from build123d import *

# Parameters (mm, degrees)
SKETCH2_R           = 7
SKETCH2_R_2         = 4
BOSS_EXTRUDE1_DEPTH = 2
SKETCH3_R           = 6.5
SKETCH3_R_2         = 4.5
CUT_EXTRUDE1_DEPTH  = 0.25
FILLET1_R           = 0.25
CHAMFER1_SIZE       = 0.125


with BuildPart() as part:
    # Sketch2 → Boss-Extrude1 (new body, symmetric)
    with BuildSketch(Plane(origin=(0, 0, 0), x_dir=(1, 0, 0), z_dir=(0, 1, 0))):
        Circle(SKETCH2_R)
        Circle(SKETCH2_R_2, mode=Mode.SUBTRACT)
    extrude(amount=BOSS_EXTRUDE1_DEPTH, both=True)

    # Sketch3 → Cut-Extrude1 (cut)
    with BuildSketch(Plane(origin=(0, 2, 0), x_dir=(1, 0, 0), z_dir=(0, 1, 0))):
        Circle(SKETCH3_R)
        Circle(SKETCH3_R_2, mode=Mode.SUBTRACT)
    cut_extrude1 = extrude(amount=-CUT_EXTRUDE1_DEPTH, mode=Mode.SUBTRACT)

    # Mirror1: Cut-Extrude1 across plane
    add(cut_extrude1.mirror(Plane.ZX), mode=Mode.SUBTRACT)

    # Fillet1
    fillet1_edges = [part.edges().sort_by_distance(p)[0] for p in [
        (-7, -2, 0),
        (-7, 2, 0),
    ]]
    fillet(fillet1_edges, radius=FILLET1_R)

    # Chamfer1
    chamfer1_edges = [part.edges().sort_by_distance(p)[0] for p in [
        (-4, -2, 0),
        (-4, 2, 0),
    ]]
    chamfer(chamfer1_edges, length=CHAMFER1_SIZE)


solid = part.part
Design review of the part built by this model. Coordinates are the model's own, in mm. A direction names the side the tool comes from. Coordinates: 2 decimals unless noted, no trailing zeros. Loops run counter-clockwise (first coordinate to the right, second up) from the corner with the lowest first, then second, coordinate; pieces in that order, holes last. Notation, with made-up numbers: (75.5, 25) -> (115.5, 25) arc R17 ccw to (115.5, 51) -> close; hole circle Ø5 at (32.25, -2.75). An arc over 180 degrees is marked (long way). Use a Markdown table: item, result. Add a question column.
Item 1: Wall thickness on L1, parallel to Z at x = 0, y = -0.45; L2, parallel to Z at x = 0, y = -1.85; L3, parallel to Z at x = 0, y = 1.9 (3 decimals): over which ranges is each line inside the solid? List them lowest first. Write a range as from..to.
Item 2: Machinability: for faces 3 (the flat face through (-4.42, 1.75, -1.54)), 4 (the cylindrical face through (-0.867, -0.026, 3.905)), which of the approach directions +Z, -Z, +X, -X, +Y, -Y give a long, thin tool a straight path to every point of the face, cutting with its end or side? Answer none if there is none.
Item 3: We need section C-C, the plane y = -1. Write out the cut boundary in (x, z).
Item 4: The part is to be moulded in two halves that separate along X. For faces 1 (the cylindrical face through (6.466, 0.024, 2.681)), 2 (the flat face through (-4.42, -1.75, -1.54)), say which applies: +X half, -X half, draft (parallel to the pull), parting line (faces both ways), or undercut.
Item 5: Clearance check with flat-ended pins moving along their axes: P1, Ø4, axis at x = 2, z = 0.5, coming from the -Y side; P2, Ø2, axis at y = 1.5, z = 2.5, coming from the +X side; P3, Ø1.5, axis at y = -0.5, z = -3, coming from the -X side. State where each tip first meets the part, or that it passes through.
Numbers:
| question | item | result |
|---|---|---|
| 1 | L1 | z = -7..-4, 4..7 |
| 1 | L2 | z = -6.98..-6.5, -4.5..-4, 4..4.5, 6.5..6.98 |
| 1 | L3 | z = -6.95..-6.5, -4.5..-4.025, 4.025..4.5, 6.5..6.95 |
| 2 | face 3 | +Y |
| 2 | face 4 | +Y, -Y |
| 3 | outline | circle Ø14 at (0, 0); hole circle Ø8 at (0, 0) |
| 4 | face 1 | parting line |
| 4 | face 2 | undercut |
| 5 | P1 | stops at y = -1.94 |
| 5 | P2 | stops at x = 6.84 |
| 5 | P3 | stops at x = -6.63 |
